```python
from build123d import *

# Parameters (mm, degrees)
SKETCH1_W                 = 25.4
SKETCH1_H                 = 12.7
SKETCH1_H_2               = 63.5
BOSS_EXTRUDE1_DEPTH       = 33.3756
CUT_EXTRUDE2_DEPTH        = 57.663045059
CUT_EXTRUDE2_DEPTH_BACK   = 57.663045059
BOSS_EXTRUDE2_REACH       = 63.744
SKETCH1_5_W               = 25.4
SKETCH1_5_H               = 12.7
SKETCH7_W                 = 25.4
SKETCH7_H                 = 3.175
BOSS_EXTRUDE3_DEPTH       = 12.7
FILLET1_R                 = 6.35
BOSS_EXTRUDE4_START       = -37.680553771
BOSS_EXTRUDE4_OUTLINE_R   = 5.08
BOSS_EXTRUDE4_DEPTH       = 16.680553771
BOSS_EXTRUDE4_START_2     = 37.680553771
BOSS_EXTRUDE4_2_OUTLINE_R = 5.08
BOSS_EXTRUDE4_2_DEPTH     = 2.722363995
BOSS_EXTRUDE4_START_3     = 37.711420882
BOSS_EXTRUDE4_3_OUTLINE_W = 14
BOSS_EXTRUDE4_3_OUTLINE_H = 14
BOSS_EXTRUDE4_3_DEPTH     = 3.288579118
CUT_EXTRUDE4_START        = -15.875
SKETCH8_3_R               = 5.715
SKETCH8_3_R_2             = 5.08
CUT_EXTRUDE4_DEPTH        = 15.875


with BuildPart() as part:
    # Sketch1 → Boss-Extrude1 (new body)
    with BuildSketch(Plane(origin=(0, 0, 0), x_dir=(1, 0, 0), z_dir=(0, 1, 0))):
        with Locations((0, -31.75)):
            Rectangle(SKETCH1_W, SKETCH1_H)
        with Locations((0, 6.35)):
            Rectangle(SKETCH1_W, SKETCH1_H_2)
    extrude(amount=BOSS_EXTRUDE1_DEPTH)

    # Sketch4 → Cut-Extrude2 (cut, two sides: drawn at the far end of the back side and taken through both)
    with BuildSketch(Plane(origin=(12.7, 0, 0), x_dir=(0, 0, -1), z_dir=(1, 0, 0)).offset(-CUT_EXTRUDE2_DEPTH_BACK)):
        Polygon((38.1, 33.3756), (-38.1, 33.3756), (-38.1, 12.957871537), align=None)
    extrude(amount=CUT_EXTRUDE2_DEPTH + CUT_EXTRUDE2_DEPTH_BACK, mode=Mode.SUBTRACT)

    # Boss-Extrude2: from a plane face, 63.744 long prism both ways, kept between that surface and its translate by the depth
    boss_extrude2_start = Plane(origin=(-12.7, 12.957871537, 38.1), z_dir=(0, -0.9659258262890681, -0.2588190451025217)) * Box(256.976, 256.976, 128.488, align=(Align.CENTER, Align.CENTER, Align.MIN), mode=Mode.PRIVATE)
    boss_extrude2_end = Plane(origin=(-12.7, 22.482871537, 38.1), z_dir=(0, -0.9659258262890681, -0.2588190451025217)) * Box(256.976, 256.976, 128.488, align=(Align.CENTER, Align.CENTER, Align.MIN), mode=Mode.PRIVATE)
    # Sketch1_5 → Boss-Extrude2 (add, from a surface)
    with BuildSketch(Plane(origin=(0, 0, 0), x_dir=(1, 0, 0), z_dir=(0, 1, 0)), mode=Mode.PRIVATE) as boss_extrude2_sk1:
        with Locations((0, -31.75)):
            Rectangle(SKETCH1_5_W, SKETCH1_5_H)
    boss_extrude2_tool1 = extrude(boss_extrude2_sk1.sketch, amount=BOSS_EXTRUDE2_REACH, both=True, mode=Mode.PRIVATE)
    add(((boss_extrude2_tool1 - boss_extrude2_start) & boss_extrude2_end).solids().sort_by_distance((0, 21.123326, 31.75))[0])

    # Sketch7 → Boss-Extrude3 (add, along a direction that is not the sketch's normal)
    with BuildSketch(Plane(origin=(0, 0, 25.4), x_dir=(-1, 0, 0), z_dir=(0, 0, -1))):
        with Locations((0, 24.298326281)):
            Rectangle(SKETCH7_W, SKETCH7_H)
    extrude(amount=BOSS_EXTRUDE3_DEPTH, dir=(0, 0.2588190451025216, -0.965925826289068))

    # Fillet1
    fillet1_edges = [part.edges().sort_by_distance(p)[0] for p in [
        (-12.7, 16.6878, -38.1),
        (-12.7, 11.241435768, 38.1),
        (12.7, 16.6878, -38.1),
        (12.7, 11.241435768, 38.1),
    ]]
    fillet(fillet1_edges, radius=FILLET1_R)

    # Boss-Extrude4: read off the stored shape, not the designer's step
    # Boss-Extrude4 outline → Boss-Extrude4 (add)
    with BuildSketch(Plane.XZ.offset(BOSS_EXTRUDE4_START)):
        Circle(BOSS_EXTRUDE4_OUTLINE_R)
    extrude(amount=BOSS_EXTRUDE4_DEPTH)

    # Boss-Extrude4 2 outline → Boss-Extrude4 2 (add)
    with BuildSketch(Plane(origin=(0, 0, 0), x_dir=(1, 0, 0), z_dir=(0, 1, 0)).offset(BOSS_EXTRUDE4_START_2)):
        Circle(BOSS_EXTRUDE4_2_OUTLINE_R)
    extrude(amount=BOSS_EXTRUDE4_2_DEPTH)

    # Boss-Extrude4 3 outline → Boss-Extrude4 3 (cut)
    with BuildSketch(Plane(origin=(0, 0, 0), x_dir=(1, 0, 0), z_dir=(0, 0.965925826289068, 0.258819045102522)).offset(BOSS_EXTRUDE4_START_3)):
        with Locations((0, 10)):
            Rectangle(BOSS_EXTRUDE4_3_OUTLINE_W, BOSS_EXTRUDE4_3_OUTLINE_H)
    extrude(amount=BOSS_EXTRUDE4_3_DEPTH, mode=Mode.SUBTRACT)

    # Sketch8_3 → Cut-Extrude4 (cut)
    # profile 1 of 2: a face of its own
    with BuildSketch(Plane.XZ.offset(CUT_EXTRUDE4_START)):
        with Locations(Location((0, 0, 0), (0, 0, 270))):
            Circle(SKETCH8_3_R)
        with Locations(Location((0, 0, 0), (0, 0, 90))):
            Circle(SKETCH8_3_R_2, mode=Mode.SUBTRACT)
    # profile 2 of 2: a face of its own
    with BuildSketch(Plane.XZ.offset(CUT_EXTRUDE4_START)):
        with Locations(Location((0, 0, 0), (0, 0, 90))):
            Circle(SKETCH8_3_R_2)
    extrude(amount=CUT_EXTRUDE4_DEPTH, mode=Mode.SUBTRACT)


solid = part.part
```
The model under review builds one solid part; all positions refer to its coordinate system, in mm. A direction names the side the tool comes from. Coordinates: 2 decimals unless noted, no trailing zeros. Order: outer loops, then holes, each group sorted by start corner. A loop starts at its lowest first (then second) coordinate and runs counter-clockwise, first axis right, second up. Notation, with made-up numbers: (-0.5, 88) -> (12.5, 88) arc R25 ccw to (12.5, 100) -> close; hole circle Ø3 at (87, -38.5). An arc over 180 degrees is marked (long way). Answer in a Markdown table with one row per item. Add a question column.
Item 1: We need section C-C on z = 2. Write out the cut boundary in (x, y) (3 decimals), plus the area to 3 significant figures.
Item 2: We need section A-A on y = 3.5. Write out the cut boundary in (x, z) (3 decimals), plus the area to 3 significant figures.
Item 3: Clearance check with flat-ended pins moving along their axes: pin 1 (12 mm diameter, centred on x = 3.5, z = 30, fed in from -Y); pin 2 (4 mm diameter, centred on x = -10, z = -3, fed in from +Y). State where each tip first meets the part, or that it passes through.
Item 4: We need section B-B on z = 22. Write out the cut boundary in (x, y).
Item 5: We need section D-D on x = -1. Write out the cut boundary in (y, z) (3 decimals).
Item 6: To check wall thickness, follow probe 1 along X at (y, z) = (12, 0) (3 decimals); probe 2 along Y at (x, z) = (1.5, 25); probe 3 along Y at (x, z) = (7.75, 21.5). State the ranges of each line that lie inside material, in increasing order.
Item 7: Mouldability with a two-part tool opening along Z and no side actions: class faces 1 (the flat face through (0, 11, 38.1)), 2 (the flat face through (0, 28, 13.133)), 3 (the flat face through (-6, 0, -1)), 4 (the flat face through (0, 20, 25.4)) as +Z half, -Z half, draft (parallel to the pull), parting line (faces both ways), or undercut.
Item 8: Machinability: for faces 5 (the flat face through (0.18, 24.33, 19.35)), 6 (the cylindrical face through (4.845, 30.958, -1.526)), 7 (the flat face through (0, 16, -38.1)), 8 (the flat face through (-12.7, 12, 0)), 9 (the flat face through (0, 15.875, 0)), which of the approach directions +Z, -Z, +X, -X, +Y, -Y give a long, thin tool a straight path to every point of the face, cutting with its end or side? Answer none if there is none.
Final values:
| question | item | result |
|---|---|---|
| 1 | outline | (-12.7, 0) -> (-5.354, 0) -> (-5.354, 15.875) -> (5.354, 15.875) -> (5.354, 0) -> (12.7, 0) -> (12.7, 22.631) -> (4.67, 22.631) -> (4.67, 38.506) -> (-4.67, 38.506) -> (-4.67, 22.631) -> (-12.7, 22.631) -> close |
| 1 | area | 553 mm2 |
| 2 | outline | (-12.7, -31.75) arc R6.35 ccw to (-6.35, -38.1) -> (6.35, -38.1) arc R6.35 ccw to (12.7, -31.75) -> (12.7, 31.75) arc R6.35 ccw to (6.35, 38.1) -> (-6.35, 38.1) arc R6.35 ccw to (-12.7, 31.75) -> close; hole circle Ø11.43 at (0, 0) |
| 2 | area | 1,800 mm2 |
| 3 | pin 1 | stops at y = 0 |
| 3 | pin 2 | stops at y = 24.51 |
| 4 | outline | (-12.7, 0) -> (12.7, 0) -> (12.7, 17.27) -> (-12.7, 17.27) -> close; (-12.7, 23.62) -> (12.7, 23.62) -> (12.7, 26.8) -> (-12.7, 26.8) -> close |
| 5 | outline | (0, -38.1) -> (33.376, -38.1) -> (24.501, -4.981) -> (40.376, -4.981) -> (37.707, 4.981) -> (21.832, 4.981) -> (16.361, 25.4) -> (22.711, 25.4) -> (25.998, 13.133) -> (29.173, 13.133) -> (22.483, 38.1) -> (0, 38.1) -> (0, 5.627) -> (15.875, 5.627) -> (15.875, -5.627) -> (0, -5.627) -> close |
| 6 | probe 1 | x = -12.7 to -5.715, 5.715 to 12.7 |
| 6 | probe 2 | y = 0 to 16.47, 22.82 to 25.99 |
| 6 | probe 3 | y = 0 to 17.41, 23.76 to 26.93 |
| 7 | face 1 | +Z half |
| 7 | face 2 | undercut |
| 7 | face 3 | draft |
| 7 | face 4 | undercut |
| 8 | face 5 | +X, -X |
| 8 | face 6 | +Y |
| 8 | face 7 | -Z, +X, -X, +Y, -Y |
| 8 | face 8 | +Z, -Z, -X, +Y, -Y |
| 8 | face 9 | -Y |
